Could you check a few things on this drawing? It's one solid part, dimensions in mm from its lowest x, y, z. Coordinates: 2 decimals unless noted, no trailing zeros. Write each loop counter-clockwise with the first axis right and the second up, starting at its lowest first coordinate (ties: lowest second). Pieces come first, ordered by that corner, then holes. Notation, with made-up numbers: M -30,14 L 14,14 A16 ccw 14,19 Z; hole C -13,-32.5 d2. An arc over 180 degrees is marked long. Use a Markdown table: item, result.
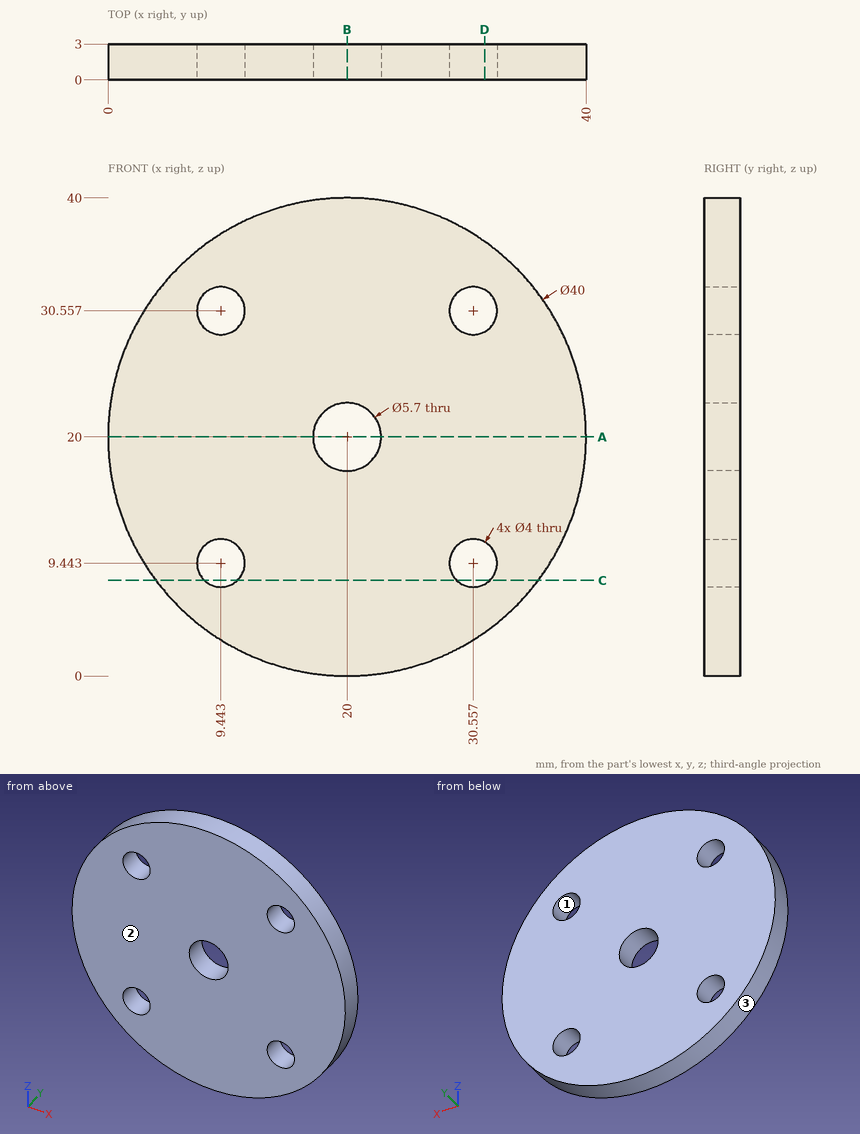
1. We'd pull the mould along Z, two halves only. Please class the marked faces 1, 2 and 3: +Z half, -Z half, draft (parallel to the pull), parting line (faces both ways), or undercut.
Answers follow:
| item | result |
|---|---|
| face 1 | undercut |
| face 2 | draft |
| face 3 | parting line |
2. Suppose I cut it at B-B on x = 20. Write out the boundary of the cut face in (y, z).
Answers follow:
| item | result |
|---|---|
| outline | M 0,0 L 3,0 L 3,17.15 L 0,17.15 Z; M 0,22.85 L 3,22.85 L 3,40 L 0,40 Z |
3. Suppose I cut it at C-C on z = 8. Write out the boundary of the cut face in (x, y).
Answers follow:
| item | result |
|---|---|
| outline | M 4,0 L 8.06,0 L 8.06,3 L 4,3 Z; M 10.83,0 L 29.17,0 L 29.17,3 L 10.83,3 Z; M 31.94,0 L 36,0 L 36,3 L 31.94,3 Z |
4. I need wall thicknesses on probe 1 along Z at (x, y) = (32, 1.85); probe 2 along Z at (x, y) = (10, 0.7); probe 3 along X at (y, z) = (1.15, 30.5). Which ranges of each line are inside material? Lowest first, please.
Answers follow:
| item | result |
|---|---|
| probe 1 | z = 4 to 8.06, 10.83 to 29.17, 31.94 to 36 |
| probe 2 | z = 2.68 to 7.52, 11.36 to 28.64, 32.48 to 37.32 |
| probe 3 | x = 2.98 to 7.44, 11.44 to 28.56, 32.56 to 37.02 |
5. Suppose I cut it at D-D on x = 31.5. Write out the boundary of the cut face in (y, z), and give its area (3 significant figures).
Answers follow:
| item | result |
|---|---|
| outline | M 0,3.64 L 3,3.64 L 3,7.68 L 0,7.68 Z; M 0,11.21 L 3,11.21 L 3,28.79 L 0,28.79 Z; M 0,32.32 L 3,32.32 L 3,36.36 L 0,36.36 Z |
| area | 77.0 mm2 |
6. Suppose I cut it at A-A on z = 20. Write out the boundary of the cut face in (x, y).
Answers follow:
| item | result |
|---|---|
| outline | M 0,0 L 17.15,0 L 17.15,3 L 0,3 Z; M 22.85,0 L 40,0 L 40,3 L 22.85,3 Z |
7. Will this pin go through, and if not, where does the flat tip stop? pin 1 Ø1.5 at (y, z) = (2.5, 11) entering from +X.
Answers follow:
| item | result |
|---|---|
| pin 1 | stops at x = 38.22 |
